Autodesk Inventor part; units mm, degrees
ref_plane "Work Plane1" through (-24, -44, 0) normal (0, -1, 0) x (1, 0, 0)
ref_plane "YZ Plane" through (0, 0, 0) normal (1, 0, 0) x (0, 1, 0)
ref_plane "XZ Plane" through (0, 0, 0) normal (0, 1, 0) x (-1, 0, 0)
sketch "Sketch1" plane through (0, 0, 0) normal (0, 0, 1) x (1, 0, 0)
  arc A0 (24, 0) -> (-24, 0) centre (0, 0) ccw
  line L0 (-24, 0) -> (-24, -44)
  line L1 (24, 0) -> (24, -44)
  dimension "d0" = 48
  dimension "d1" = 44
ref_plane "Work Plane1" through (-24, -44, 0) normal (0, -1, 0) x (1, 0, 0)
sketch "Sketch2" plane through (-24, -44, 0) normal (0, -1, 0) x (1, 0, 0)
  circle A0 centre (0, 0) radius 4
  point P0 (24, 0)
  dimension "d2" = 8
sweep "Колебание1" add profiles "Sketch2" path "Sketch1"
thread "Резьба1"
thread "Резьба2"
chamfer "Фаска1" distance 1 angle 45 2 edges at (28, -44, 0) (-28, -44, 0)
equation "\"d0\" = D + d_"
equation "\"d1\" = -d_ + H_ - 0.5 * D"
equation "\"d2\" = d_"
equation "\"d4\" = l_"
equation "\"d11\" = l_"
equation "\"D\" = 40"
equation "\"A_\" = 48"
equation "\"H_\" = 72"
equation "\"d_\" = 8"
equation "\"l_\" = 34"
properties part number "Скоба 40 ГОСТ 24137-80" material "Сталь, мягкая"
The model under review builds one solid part; all positions refer to its coordinate system, in mm. Round coordinates to 2 decimals unless told otherwise and drop trailing zeros. Write each loop counter-clockwise with the first axis right and the second up, starting at its lowest first coordinate (ties: lowest second). Pieces come first, ordered by that corner, then holes. Notation, with made-up numbers: (-30, 44) - (-19, 44) arc R22 cw to (-19, 61) - close; hole circle Ø4 at (-35.75, -20.75). An arc over 180 degrees is marked (long way). One line per question, with ' | ' between items.
Item 1: To check wall thickness, follow probe 1 along X at (y, z) = (-22, 0.25); probe 2 along X at (y, z) = (-39, -2.5); probe 3 along Y at (x, z) = (16.5, -3). State the ranges of each line that lie inside material, in increasing order.
Resolved:
probe 1: x = -27.99 to -20.01, 20.01 to 27.99 | probe 2: x = -27.12 to -20.88, 20.88 to 27.12 | probe 3: y = 13.56 to 20.92
Item 2: Add section B-B, the plane z = 0. Give the boundary of the cut face in (x, y), then the cut area to 3 significant figures.
Resolved:
outline: (-28, -43) - (-27, -44) - (-21, -44) - (-20, -43) - (-20, 0) arc R20 cw to (20, 0) - (20, -43) - (21, -44) - (27, -44) - (28, -43) - (28, 0) arc R28 ccw to (-28, 0) - close | area: 1,310 mm2
Item 3: Add section A-A, the plane y = -22.5. Give the boundary of the cut face in (x, z), then the cut area to 3 significant figures.
Resolved:
outline: circle Ø8 at (-24, 0); circle Ø8 at (24, 0) | area: 101 mm2
Item 4: For P1, Ø10, axis at x = 11.5, y = -28, coming from the +Z side; P2, Ø1.5, axis at y = -12, z = -2, coming from the -X side; P3, Ø1.5, axis at x = -21.5, y = -21.5, coming from the -Z side, all flat-tipped, find the tip position at first contact; note any pin that passes through.
Resolved:
P1: passes through | P2: stops at x = -27.8 | P3: stops at z = -3.6
Item 5: The part is to be moulded in two halves that separate along X. For faces 1 (the face through (-27.2, -21.8, -2.4)), 2 (the face through (24, -44, 0)), 3 (the face through (27.2, -21.2, -2.4)), say which applies: pulls with the +X half, pulls with the -X half, needs draft (parallel to the pull), parting line crosses it, or undercut.
Resolved:
face 1: undercut | face 2: needs draft | face 3: undercut
